Verification items for the finished model (mm, model axes). Face numbers are marked on the shaded views. A direction names the side the tool comes from. Round coordinates to 2 decimals unless told otherwise and drop trailing zeros. Loops run counter-clockwise (first coordinate to the right, second up) from the corner with the lowest first, then second, coordinate; pieces in that order, holes last. Notation, with made-up numbers: (-33, 68.5) -> (-25, 68.5) arc R18 cw to (-25, 86.5) -> close; hole circle Ø3 at (80, 50). An arc over 180 degrees is marked (long way). Write item = value, one per line.
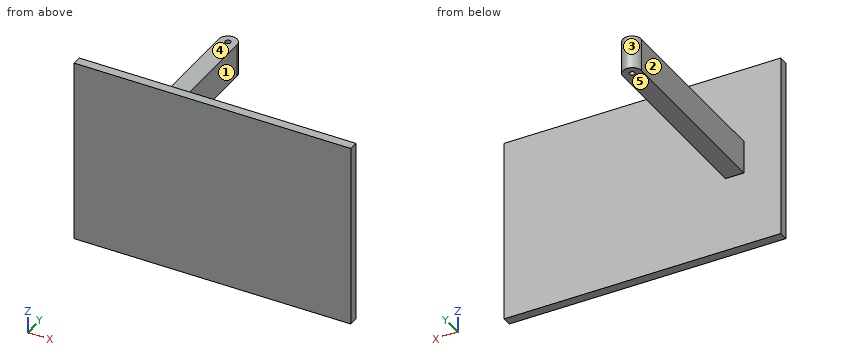
```python
from build123d import *

# Parameters (mm, degrees)
BOSS_EXTRUDE1_DEPTH = 1.27
SKETCH2_W           = 2.54
SKETCH2_H           = 4.572
BOSS_EXTRUDE2_DEPTH = 25.4
SKETCH3_R           = 1.27
BOSS_EXTRUDE3_DEPTH = 4.572
SKETCH4_R           = 0.381
CUT_EXTRUDE1_DEPTH  = 4.572


with BuildPart() as part:
    # Sketch1 → Boss-Extrude1 (new body)
    with BuildSketch(Plane(origin=(0, 0, 0), x_dir=(1, 0, 0), z_dir=(0, 1, 0))):
        Polygon((-12.7, 12.7), (12.7, 12.7), (25.4, 12.7), (25.4, -12.7), (12.7, -12.7), (-12.7, -12.7), align=None)
    extrude(amount=BOSS_EXTRUDE1_DEPTH)

    # Sketch2 → Boss-Extrude2 (add)
    with BuildSketch(Plane(origin=(0, 1.27, 0), x_dir=(1, 0, 0), z_dir=(0, 1, 0))):
        with Locations((-6.35, 0)):
            Rectangle(SKETCH2_W, SKETCH2_H)
    extrude(amount=BOSS_EXTRUDE2_DEPTH)

    # Sketch3 → Boss-Extrude3 (add)
    with BuildSketch(Plane.XY.offset(2.286)):
        with Locations((-6.35, 26.67)):
            Circle(SKETCH3_R)
    extrude(amount=-BOSS_EXTRUDE3_DEPTH)

    # Sketch4 → Cut-Extrude1 (cut)
    with BuildSketch(Plane.XY.offset(2.286)):
        with Locations((-6.35, 26.67)):
            Circle(SKETCH4_R)
    extrude(amount=-CUT_EXTRUDE1_DEPTH, mode=Mode.SUBTRACT)


solid = part.part
```
(1) Sectioned sample at C-C, the plane x = 0. Record the cut outline in (y, z), and give its area (3 significant figures).
Filled sheet:
outline = (0, -12.7) -> (1.27, -12.7) -> (1.27, 12.7) -> (0, 12.7) -> close
area = 32.3 mm2
(2) Go/stop test with flat-tipped pins: pin 1 Ø6 at (x, y) = (-2.5, 21) entering from -Z; pin 2 Ø5 at (y, z) = (10, 0.5) entering from -X; pin 3 Ø2 at (x, y) = (-5.5, 18) entering from +Z; pin 4 Ø1 at (x, z) = (7, 8) entering from -Y. Record where each tip stops, or that it passes through.
Filled sheet:
pin_1 = -2.29
pin_2 = -7.62
pin_3 = 2.29
pin_4 = 0
(3) Sectioned sample at B-B, the plane y = 6.5. Record the cut outline in (x, z).
Filled sheet:
outline = (-7.62, -2.29) -> (-5.08, -2.29) -> (-5.08, 2.29) -> (-7.62, 2.29) -> close
(4) Material ranges on probe 1 along Y at (x, z) = (-6.35, -0.9); probe 2 along X at (y, z) = (26.67, 0.35); probe 3 along Y at (x, z) = (17, -2.5), recorded low to high. Write a range as from..to.
Filled sheet:
probe_1 = 0..26.29, 27.05..27.94
probe_2 = -7.62..-6.73, -5.97..-5.08
probe_3 = 0..1.27
(5) Set-up check for the marked faces 1, 2, 3, 4 and 5: record each of +Z, -Z, +X, -X, +Y, -Y from which the full face is reachable in a straight line by a thin tool's end or side.
Filled sheet:
face_1 = +Z, -Z, +X, +Y
face_2 = +Z, -Z, -X, +Y
face_3 = +Z, -Z, +Y
face_4 = +Z, +X, -X, +Y
face_5 = -Z, +X, -X, +Y
(6) Sectioned sample at A-A, the plane z = 1. Record the cut outline in (x, y), and give its area (3 significant figures).
Filled sheet:
outline = (-12.7, 0) -> (25.4, 0) -> (25.4, 1.27) -> (-5.08, 1.27) -> (-5.08, 26.67) arc R1.27 ccw to (-7.62, 26.67) -> (-7.62, 1.27) -> (-12.7, 1.27) -> close; hole circle Ø0.76 at (-6.35, 26.67)
area = 115 mm2
